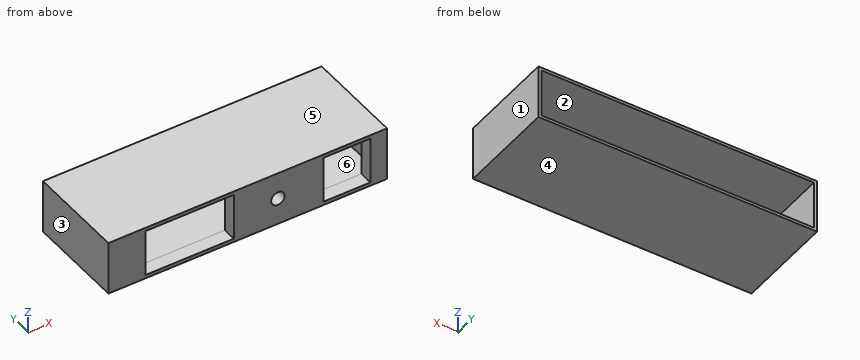
```python
from build123d import *

# Parameters (mm, degrees)
SKETCH1_W           = 104.14
SKETCH1_H           = 20.193
BOSS_EXTRUDE1_DEPTH = 5.08
SKETCH2_W           = 104.14
SKETCH2_H           = 20.193
SKETCH2_W_2         = 101.854
SKETCH2_H_2         = 18.034
BOSS_EXTRUDE2_DEPTH = 32.004
SKETCH3_R           = 2.54
SKETCH3_W           = 33.02
SKETCH3_H           = 17.526
SKETCH3_W_2         = 17.526
CUT_EXTRUDE1_DEPTH  = 32.004


with BuildPart() as part:
    # Sketch1 → Boss-Extrude1 (new body)
    with BuildSketch(Plane(origin=(0, 0, 0), x_dir=(1, 0, 0), z_dir=(0, 1, 0))):
        Rectangle(SKETCH1_W, SKETCH1_H)
    extrude(amount=BOSS_EXTRUDE1_DEPTH)

    # Sketch2 → Boss-Extrude2 (add)
    with BuildSketch(Plane(origin=(0, 5.08, 0), x_dir=(1, 0, 0), z_dir=(0, 1, 0))):
        Rectangle(SKETCH2_W, SKETCH2_H)
        Rectangle(SKETCH2_W_2, SKETCH2_H_2, mode=Mode.SUBTRACT)
    extrude(amount=BOSS_EXTRUDE2_DEPTH)

    # Sketch3 → Cut-Extrude1 (cut)
    with BuildSketch(Plane(origin=(0, 5.08, 0), x_dir=(1, 0, 0), z_dir=(0, 1, 0))):
        with Locations(Location((11.303, 0, 0), (0, 0, 270))):
            Circle(SKETCH3_R)
        with Locations((-21.717, 0)):
            Rectangle(SKETCH3_W, SKETCH3_H)
        with Locations((37.084, 0)):
            Rectangle(SKETCH3_W_2, SKETCH3_H)
    extrude(amount=-CUT_EXTRUDE1_DEPTH, mode=Mode.SUBTRACT)


solid = part.part
```
Source: CAD feature listing. Evaluate the final solid. Frame: model axes, mm. Face numbers are marked on the shaded views. A direction names the side the tool comes from. Coordinates: 2 decimals unless noted, no trailing zeros. Loops run counter-clockwise (first coordinate to the right, second up) from the corner with the lowest first, then second, coordinate; pieces in that order, holes last. Notation, with made-up numbers: M -5,84 L 53,84 A20 cw 53,95 Z; hole C -19.5,6 d10. An arc over 180 degrees is marked long. Use a Markdown table: item, result. Add a question column.
Q1. Section query B-B, the plane y = 15. Return loops of the section in (x, z).
Q2. First-contact query: pin 1 (3 mm diameter, centred on x = 11.303, z = 0, fed in from +Y). Flat tip, straight axial feed; report the tip coordinate or a pass-through.
Q3. Material intervals for L1, parallel to X at y = 4, z = -7.5; L2, parallel to X at y = 2.65, z = 0; L3, parallel to Z at x = -33.5, y = 27, sorted ascending.
Q4. Section query C-C, the plane x = -21. Return loops of the section in (y, z), and give its area (3 significant figures).
Q5. Access query for the marked faces 5 and 6. Directions: +Z, -Z, +X, -X, +Y, -Y. A direction counts if a zero-diameter tool reaches every point of the face in a straight line with its end or side. Return the directions, or none.
Q6. Section query A-A, the plane z = 3.75. Return loops of the section in (x, y), and give its area (3 significant figures).
Q7. Draft query along X for the marked faces 1, 2, 3 and 4. Return one class per face: pulls with the +X half, pulls with the -X half, needs draft (parallel to the pull), parting line crosses it, or undercut.
Q8. Section query D-D, the plane x = 3. Return loops of the section in (y, z), and give its area (3 significant figures).
Result:
| question | item | result |
|---|---|---|
| 1 | outline | M -52.07,-10.1 L 52.07,-10.1 L 52.07,10.1 L -52.07,10.1 Z; hole M -50.93,-9.02 L 50.93,-9.02 L 50.93,9.02 L -50.93,9.02 Z |
| 2 | pin 1 | passes through |
| 3 | L1 | x = -52.07 to -38.23, -5.21 to 28.32, 45.85 to 52.07 |
| 3 | L2 | x = -52.07 to -38.23, -5.21 to 8.76, 13.84 to 28.32, 45.85 to 52.07 |
| 3 | L3 | z = -10.1 to -9.02, 9.02 to 10.1 |
| 4 | outline | M 0,-10.1 L 37.08,-10.1 L 37.08,-9.02 L 5.08,-9.02 L 5.08,-8.76 L 0,-8.76 Z; M 0,8.76 L 5.08,8.76 L 5.08,9.02 L 37.08,9.02 L 37.08,10.1 L 0,10.1 Z |
| 4 | area | 82.6 mm2 |
| 5 | face 5 | +Z, +X, -X, +Y, -Y |
| 5 | face 6 | +Y |
| 6 | outline | M -52.07,0 L -38.23,0 L -38.23,5.08 L -50.93,5.08 L -50.93,37.08 L -52.07,37.08 Z; M -5.21,0 L 28.32,0 L 28.32,5.08 L -5.21,5.08 Z; M 45.85,0 L 52.07,0 L 52.07,37.08 L 50.93,37.08 L 50.93,5.08 L 45.85,5.08 Z |
| 6 | area | 345 mm2 |
| 7 | face 1 | pulls with the +X half |
| 7 | face 2 | undercut |
| 7 | face 3 | pulls with the -X half |
| 7 | face 4 | needs draft |
| 8 | outline | M 0,-10.1 L 37.08,-10.1 L 37.08,-9.02 L 5.08,-9.02 L 5.08,9.02 L 37.08,9.02 L 37.08,10.1 L 0,10.1 Z |
| 8 | area | 172 mm2 |
